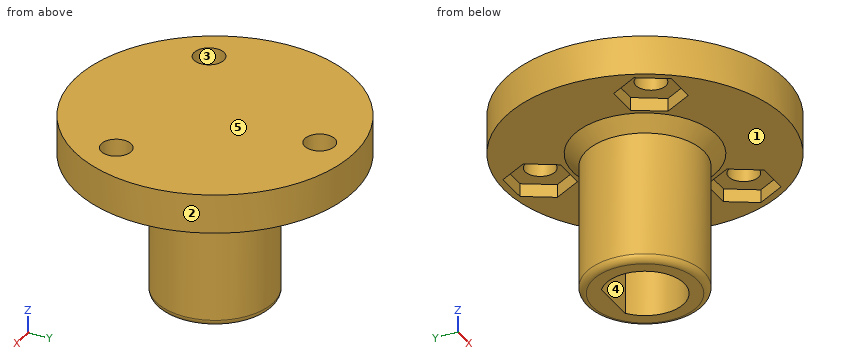
```python
from build123d import *

# Parameters (mm, degrees)
SKETCH1_R           = 4.5
BOSS_EXTRUDE1_DEPTH = 11
SKETCH2_R           = 10.75
SKETCH2_R_2         = 1.15
BOSS_EXTRUDE2_DEPTH = 3
CUT_EXTRUDE1_DEPTH  = 1
CHAMFER1_SIZE       = 1
FILLET1_R           = 0.5


with BuildPart() as part:
    # Sketch1 → Boss-Extrude1 (new body)
    with BuildSketch(Plane.XY):
        with Locations((19.925, -7)):
            Circle(SKETCH1_R)
        with BuildLine():
            Line((18.146986881, -4.583666134), (21.703013119, -4.583666134))
            ThreePointArc((21.703013119, -4.583666134), (19.925, -10), (18.146986881, -4.583666134))
        make_face(mode=Mode.SUBTRACT)
    extrude(amount=-BOSS_EXTRUDE1_DEPTH)

    # Sketch2 → Boss-Extrude2 (add)
    with BuildSketch(Plane.XY):
        with Locations((19.925, -7)):
            Circle(SKETCH2_R)
        with Locations((19.925, 1)):
            Circle(SKETCH2_R_2, mode=Mode.SUBTRACT)
        with Locations((12.99679677, -11)):
            Circle(SKETCH2_R_2, mode=Mode.SUBTRACT)
        with Locations((26.85320323, -11)):
            Circle(SKETCH2_R_2, mode=Mode.SUBTRACT)
    extrude(amount=BOSS_EXTRUDE2_DEPTH)

    # Sketch3 → Cut-Extrude1 (cut)
    with BuildSketch(Plane(origin=(0, 0, 0), x_dir=(-1, 0, 0), z_dir=(0, 0, -1))):
        Polygon((-25.583032638, -8.8), (-28.123373822, -8.8), (-29.393544415, -11), (-28.123373822, -13.2), (-25.583032638, -13.2), (-24.312862046, -11), align=None)
        Polygon((-22.465341184, 1), (-21.195170592, -1.2), (-18.654829408, -1.2), (-17.384658816, 1), (-18.654829408, 3.2), (-21.195170592, 3.2), align=None)
        Polygon((-14.266967362, -8.8), (-15.537137954, -11), (-14.266967362, -13.2), (-11.726626178, -13.2), (-10.456455585, -11), (-11.726626178, -8.8), align=None)
    extrude(amount=-CUT_EXTRUDE1_DEPTH, mode=Mode.SUBTRACT)

    # Chamfer1
    chamfer1_edges = [part.edges().sort_by_distance(p)[0] for p in [
        (15.425, -7, 0),
    ]]
    chamfer(chamfer1_edges, length=CHAMFER1_SIZE)

    # Fillet1
    fillet1_edges = [part.edges().sort_by_distance(p)[0] for p in [
        (15.425, -7, -11),
    ]]
    fillet(fillet1_edges, radius=FILLET1_R)


solid = part.part
```
Source: CAD feature listing. Evaluate the final solid. Frame: model axes, mm. Face numbers are marked on the shaded views. A direction names the side the tool comes from. Round coordinates to 2 decimals unless told otherwise and drop trailing zeros. Loops run counter-clockwise (first coordinate to the right, second up) from the corner with the lowest first, then second, coordinate; pieces in that order, holes last.
1. Section query A-A on y = -7. Output: boundary loops of the cut face in (x, z) (3 decimals), and give its area (3 significant figures).
2. Access query for the marked faces 4 and 5. Directions: +Z, -Z, +X, -X, +Y, -Y. A direction counts if a zero-diameter tool reaches every point of the face in a straight line with its end or side. Return the directions, or none.
3. Mould query, pull axis X, two halves, no side actions, for the marked faces 1, 2 and 3. Classes: released by +X, released by -X, zero draft, split by the parting line, or undercut.
4. Section query B-B on x = 12.5. Output: boundary loops of the cut face in (y, z).
5. Section query D-D on z = -8.5. Output: boundary loops of the cut face in (x, y) (3 decimals).
6. Contact query for flat-ended pins moving along their axis: pin 1 (1.5 mm diameter, centred on x = 16, z = -0.5, fed in from +Y); pin 2 (1.3 mm diameter, centred on x = 27, y = -11, fed in from -Z); pin 3 (5 mm diameter, centred on x = 11.5, z = -0.5, fed in from -Y); pin 4 (3 mm diameter, centred on x = 26.85, y = -11, fed in from -Z). Output: stop coordinate, or through.
7. Section query C-C on z = 1.5. Output: boundary loops of the cut face in (x, y) (3 decimals).
8. Ray query, L1, parallel to X at y = -11, z = 2.3; L2, parallel to X at y = -7.75, z = -7.25; L3, parallel to Z at x = 12, y = -12. Return the intervals inside material, ascending.
Answers below:
1. outline: (9.175, 0) - (14.425, 0) - (15.425, -1) - (15.425, -10.5) arc R0.5 ccw to (15.925, -11) - (16.925, -11) - (16.925, 0) - (22.925, 0) - (22.925, -11) - (23.925, -11) arc R0.5 ccw to (24.425, -10.5) - (24.425, -1) - (25.425, 0) - (30.675, 0) - (30.675, 3) - (9.175, 3) - close
1. area: 98.4 mm2
2. face 4: -Z
2. face 5: +Z, +X, -X, +Y, -Y
3. face 1: zero draft
3. face 2: split by the parting line
3. face 3: undercut
4. outline: (-14.77, 0) - (-13.2, 0) - (-13.2, 1) - (-12.04, 1) - (-12.04, 3) - (-14.77, 3) - close; (-9.96, 1) - (-8.8, 1) - (-8.8, 0) - (0.77, 0) - (0.77, 3) - (-9.96, 3) - close
5. outline: circle Ø9 at (19.925, -7); hole (18.147, -4.584) arc R3 ccw (long way) to (21.703, -4.584) - close
6. pin 1: stops at y = 3.21
6. pin 2: passes through
6. pin 3: stops at y = -15.94
6. pin 4: stops at z = 1
7. outline: circle Ø21.5 at (19.925, -7); hole circle Ø2.3 at (12.997, -11); hole circle Ø2.3 at (19.925, 1); hole circle Ø2.3 at (26.853, -11)
8. L1: x = 9.95 to 11.85, 14.15 to 25.7, 28 to 29.9
8. L2: x = 15.49 to 17.02, 22.83 to 24.36
8. L3: z = 1 to 3
